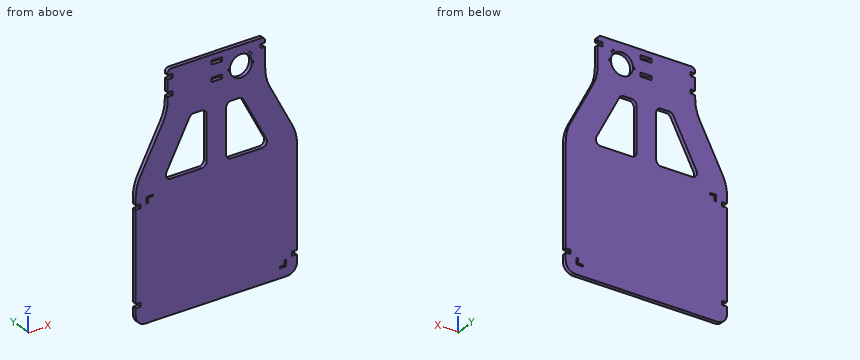
```python
from build123d import *

# Parameters (mm, degrees)
SKETCH1_W           = 22
SKETCH1_H           = 8
SKETCH1_R           = 1.75
BOSS_EXTRUDE1_DEPTH = 8


with BuildPart() as part:
    # Sketch1 → Boss-Extrude1 (new body)
    with BuildSketch(Plane(origin=(0, 0, 0), x_dir=(1, 0, 0), z_dir=(0, 1, 0))):
        with BuildLine():
            Line((-92, 0), (92, 0))
            ThreePointArc((92, 0), (97.656854249, 2.343145751), (100, 8))
            Line((100, 8), (100, 10))
            ThreePointArc((100, 10), (99.707106781, 10.707106781), (99, 11))
            Line((99, 11), (90, 11))
            Line((90, 11), (90, 19))
            Line((90, 19), (99, 19))
            ThreePointArc((99, 19), (99.707106781, 19.292893219), (100, 20))
            Line((100, 20), (100, 60.303296759))
            ThreePointArc((100, 60.303296759), (102.319800375, 79.428844756), (109.144664654, 97.445206417))
            Line((109.144664654, 97.445206417), (155.855335346, 186.554793583))
            ThreePointArc((155.855335346, 186.554793583), (162.680199625, 204.571155244), (165, 223.696703241))
            Line((165, 223.696703241), (165, 426))
            ThreePointArc((165, 426), (164.707106781, 426.707106781), (164, 427))
            Line((164, 427), (155, 427))
            Line((155, 427), (155, 435))
            Line((155, 435), (164, 435))
            ThreePointArc((164, 435), (164.707106781, 435.292893219), (165, 436))
            Line((165, 436), (165, 450))
            ThreePointArc((165, 450), (159.142135624, 464.142135624), (145, 470))
            Line((145, 470), (-145, 470))
            ThreePointArc((-145, 470), (-159.142135624, 464.142135624), (-165, 450))
            Line((-165, 450), (-165, 436))
            ThreePointArc((-165, 436), (-164.707106781, 435.292893219), (-164, 435))
            Line((-164, 435), (-155, 435))
            Line((-155, 435), (-155, 427))
            Line((-155, 427), (-164, 427))
            ThreePointArc((-164, 427), (-164.707106781, 426.707106781), (-165, 426))
            Line((-165, 426), (-165, 248))
            ThreePointArc((-165, 248), (-164.707106781, 247.292893219), (-164, 247))
            Line((-164, 247), (-155, 247))
            Line((-155, 247), (-155, 239))
            Line((-155, 239), (-164, 239))
            ThreePointArc((-164, 239), (-164.707106781, 238.707106781), (-165, 238))
            Line((-165, 238), (-165, 223.696703241))
            ThreePointArc((-165, 223.696703241), (-162.680199625, 204.571155244), (-155.855335346, 186.554793583))
            Line((-155.855335346, 186.554793583), (-109.144664654, 97.445206417))
            ThreePointArc((-109.144664654, 97.445206417), (-102.319800375, 79.428844756), (-100, 60.303296759))
            Line((-100, 60.303296759), (-100, 53))
            ThreePointArc((-100, 53), (-99.707106781, 52.292893219), (-99, 52))
            Line((-99, 52), (-90, 52))
            Line((-90, 52), (-90, 44))
            Line((-90, 44), (-99, 44))
            ThreePointArc((-99, 44), (-99.707106781, 43.707106781), (-100, 43))
            Line((-100, 43), (-100, 20))
            ThreePointArc((-100, 20), (-99.707106781, 19.292893219), (-99, 19))
            Line((-99, 19), (-90, 19))
            Line((-90, 19), (-90, 11))
            Line((-90, 11), (-99, 11))
            ThreePointArc((-99, 11), (-99.707106781, 10.707106781), (-100, 10))
            Line((-100, 10), (-100, 8))
            ThreePointArc((-100, 8), (-97.656854249, 2.343145751), (-92, 0))
        make_face()
        with BuildLine():
            Line((-55.146951484, 105.357261293), (-102.324370839, 195.357261293))
            ThreePointArc((-102.324370839, 195.357261293), (-102.023953996, 205.175548905), (-93.467453921, 210))
            Line((-93.467453921, 210), (-30, 210))
            ThreePointArc((-30, 210), (-22.928932188, 207.071067812), (-20, 200))
            Line((-20, 200), (-20, 110))
            ThreePointArc((-20, 110), (-22.928932188, 102.928932188), (-30, 100))
            Line((-30, 100), (-46.290034566, 100))
            ThreePointArc((-46.290034566, 100), (-51.465583471, 101.443499925), (-55.146951484, 105.357261293))
        make_face(mode=Mode.SUBTRACT)
        with Locations((1, 15)):
            Rectangle(SKETCH1_W, SKETCH1_H, mode=Mode.SUBTRACT)
        with Locations((1, 48)):
            Rectangle(SKETCH1_W, SKETCH1_H, mode=Mode.SUBTRACT)
        with Locations((25.26, 40)):
            Circle(SKETCH1_R, mode=Mode.SUBTRACT)
        with BuildLine():
            ThreePointArc((63.646526688, 22.110832625), (34.090097423, 55.909902577), (67.889167375, 26.353473312))
            Line((67.889167375, 26.353473312), (72.131808062, 22.110832625))
            Line((72.131808062, 22.110832625), (67.889167375, 17.868191938))
            Line((67.889167375, 17.868191938), (63.646526688, 22.110832625))
        make_face(mode=Mode.SUBTRACT)
        with Locations((74.74, 40)):
            Circle(SKETCH1_R, mode=Mode.SUBTRACT)
        with BuildLine():
            ThreePointArc((20, 200), (22.928932188, 207.071067812), (30, 210))
            Line((30, 210), (93.467453921, 210))
            ThreePointArc((93.467453921, 210), (102.023953996, 205.175548905), (102.324370839, 195.357261293))
            Line((102.324370839, 195.357261293), (55.146951484, 105.357261293))
            ThreePointArc((55.146951484, 105.357261293), (51.465583471, 101.443499925), (46.290034566, 100))
            Line((46.290034566, 100), (30, 100))
            ThreePointArc((30, 100), (22.928932188, 102.928932188), (20, 110))
            Line((20, 110), (20, 200))
        make_face(mode=Mode.SUBTRACT)
        with BuildLine():
            ThreePointArc((-140.7, 242), (-139.992893219, 241.707106781), (-139.7, 241))
            Line((-139.7, 241), (-139.7, 233))
            ThreePointArc((-139.7, 233), (-139.407106781, 232.292893219), (-138.7, 232))
            Line((-138.7, 232), (-130.7, 232))
            ThreePointArc((-130.7, 232), (-129.992893219, 231.707106781), (-129.7, 231))
            Line((-129.7, 231), (-129.7, 230))
            ThreePointArc((-129.7, 230), (-129.992893219, 229.292893219), (-130.7, 229))
            Line((-130.7, 229), (-141.7, 229))
            ThreePointArc((-141.7, 229), (-142.407106781, 229.292893219), (-142.7, 230))
            Line((-142.7, 230), (-142.7, 241))
            ThreePointArc((-142.7, 241), (-142.407106781, 241.707106781), (-141.7, 242))
            Line((-141.7, 242), (-140.7, 242))
        make_face(mode=Mode.SUBTRACT)
        with BuildLine():
            Line((129.7, 448.9), (129.7, 449.9))
            ThreePointArc((129.7, 449.9), (129.992893219, 450.607106781), (130.7, 450.9))
            Line((130.7, 450.9), (141.7, 450.9))
            ThreePointArc((141.7, 450.9), (142.407106781, 450.607106781), (142.7, 449.9))
            Line((142.7, 449.9), (142.7, 438.9))
            ThreePointArc((142.7, 438.9), (142.407106781, 438.192893219), (141.7, 437.9))
            Line((141.7, 437.9), (140.7, 437.9))
            ThreePointArc((140.7, 437.9), (139.992893219, 438.192893219), (139.7, 438.9))
            Line((139.7, 438.9), (139.7, 446.9))
            ThreePointArc((139.7, 446.9), (139.407106781, 447.607106781), (138.7, 447.9))
            Line((138.7, 447.9), (130.7, 447.9))
            ThreePointArc((130.7, 447.9), (129.992893219, 448.192893219), (129.7, 448.9))
        make_face(mode=Mode.SUBTRACT)
    extrude(amount=BOSS_EXTRUDE1_DEPTH)


solid = part.part
```
The listing builds one solid part. Answer for the finished solid, in the listing's coordinates (mm). Give positions to 0.01 mm unless a question says otherwise; leave off trailing zeros. Write each loop counter-clockwise with the first axis right and the second up, starting at its lowest first coordinate (ties: lowest second). Pieces come first, ordered by that corner, then holes. Notation, with made-up numbers: (0.5, -7) -> (29.5, -7) arc R26 cw to (29.5, 30) -> close; hole circle Ø11 at (38, 22.25). An arc over 180 degrees is marked (long way). Write item = value, one per line. Start each with the question number.
1) Straight lines are drawn through the part: line 1 along X through (y, z) = (3, -40); line 2 along Z through (x, y) = (74.74, 2.5); line 3 along Z through (x, y) = (25.26, 3.75). For each, find the intervals that lie inside material, in ascending order.
2) The part is cut by section A-A, the plane x = 83.5. Determine the outline of the cut face in (y, z).
3) Each of these flat-tipped pins is pushed along its axis until it touches: pin 1 (2.5 mm diameter, centred on x = -158, y = 2.5, fed in from +Z); pin 2 (4 mm diameter, centred on x = 135, y = 5, fed in from +Z); pin 3 (1.1 mm diameter, centred on x = -141.5, y = 3.5, fed in from +Z). Where does it stop, or does it pass through?
4) The part is cut by section B-B, the plane y = 5.25. Count the separate pieces of the cut face and the enclosed holes in it, and give its area (3 significant figures).
Solutions:
q1.line_1 = -100 to 23.51, 27.01 to 27.5, 72.5 to 72.99, 76.49 to 100
q1.line_2 = -470 to -210, -142.73 to -41.75, -38.25 to 0
q1.line_3 = -470 to -208.81, -101.19 to -41.75, -38.25 to 0
q2.outline = (0, -470) -> (8, -470) -> (8, -210) -> (0, -210) -> close; (0, -159.45) -> (8, -159.45) -> (8, 0) -> (0, 0) -> close
q3.pin_1 = -188.31
q3.pin_2 = -142.95
q3.pin_3 = -158.12
q4.separate_pieces = 1
q4.enclosed_holes = 9
q4.area = 121,000 mm²
